Verification items for the finished model (mm, model axes). Round coordinates to 2 decimals unless told otherwise and drop trailing zeros. Loops run counter-clockwise (first coordinate to the right, second up) from the corner with the lowest first, then second, coordinate; pieces in that order, holes last. Notation, with made-up numbers: (-3, 4.25) -> (45, 4.25) arc R22 ccw to (45, 10.25) -> close; hole circle Ø9 at (-17.75, -30.75). An arc over 180 degrees is marked (long way). Use CSV: the item, a comma, the result in double quotes. Start each with the question number.
Autodesk Inventor part; units mm, degrees
ref_plane "YZ Plane" through (0, 0, 0) normal (1, 0, 0) x (0, 1, 0)
ref_plane "XZ Plane" through (0, 0, 0) normal (0, 1, 0) x (-1, 0, 0)
ref_plane "XY Plane" through (0, 0, 0) normal (0, 0, 1) x (1, 0, 0)
sketch "Sketch1" plane through (0, 0, 0) normal (0, 1, 0) x (-1, 0, 0)
  arc A0 (-2.75, 2.165064) -> (2.75, 2.165064) centre (0, 0) ccw
  line L0 (-1.9, 14.1) -> (-2.75, 2.165064)
  line L1 (1.898718, 14.098684) -> (2.75, 2.165064)
  arc A1 (1.898718, 14.098684) -> (-1.9, 14.1) centre (-0.000658, 14.05) ccw
  circle A2 centre (0, 0) radius 0.5
  line L2 (0, 0) -> (0, -10) construction
  line L3 (0, 30) -> (0, 0) construction
  arc A3 (-7.653502, 3.697825) -> (7.653343, 3.698154) centre (0, 0) ccw
  line L4 (7.653343, 3.698154) -> (6.891627, 14.376202)
  arc A4 (6.891627, 14.376202) -> (-6.892842, 14.378331) centre (-0.000658, 14.05) ccw
  line L5 (-6.892842, 14.378331) -> (-7.653502, 3.697825)
  line L6 (10, 0) -> (-10, 0)
  line L7 (-10, 0) -> (-10, 30)
  line L8 (-10, 30) -> (10, 30)
  line L9 (10, 30) -> (10, 0)
  point P0 (-8.5, 0)
  point P1 (8.5, 0)
  dimension "d0" = 1
  dimension "d9" = 1.9
  dimension "d11" = 3.5
  dimension "d34" = 10
  dimension "d42" = 5
  dimension "d43" = 20
  dimension "d44" = 30
sketch "Sketch1 outline for Extrusion6" plane through (0, 0, 0) normal (0, 1, 0) x (-1, 0, 0)
  arc A0 (-8.5, 0) -> (8.5, 0) centre (0, 0) ccw
  line L0 (-10, 0) -> (-8.5, 0)
  line L1 (8.5, 0) -> (10, 0)
  line L2 (-10, 30) -> (-10, 0)
  line L3 (10, 0) -> (10, 30)
  line L4 (10, 30) -> (-10, 30)
  arc A1 (2.75, 2.165064) -> (-2.75, 2.165064) centre (0, 0) cw
  line L5 (1.898718, 14.098684) -> (2.75, 2.165064)
  arc A2 (-1.9, 14.1) -> (1.898718, 14.098684) centre (-0.000658, 14.05) cw
  line L6 (-2.75, 2.165064) -> (-1.9, 14.1)
extrude "Extrusion6" add sketch "Sketch1 outline for Extrusion6" along normal blind 8
sketch "Sketch7" plane through (0, 0, 0) normal (0, -1, 0) x (1, 0, 0)
  arc A0 (-8.5, 0) -> (8.5, 0) centre (0, 0) ccw
  line L0 (10, 30) -> (10, 0)
  line L1 (-10, 0) -> (-10, 30)
  line L2 (-10, 0) -> (-10, 30)
  line L3 (-10, 0) -> (-7.225, -4.477653)
  line L4 (10, 0) -> (7.225, -4.477653)
  line L5 (8.5, 0) -> (10, 0)
  line L6 (-8.5, 0) -> (-10, 0)
  line L7 (-8.5, 0) -> (-10, 0)
sketch "Sketch7 outline for Extrusion7" plane through (0, 0, 0) normal (0, -1, 0) x (1, 0, 0)
  line L0 (-8.5, 0) -> (-10, 0)
  arc A0 (-7.225, -4.477653) -> (-8.5, 0) centre (0, 0) cw
  line L1 (-10, 0) -> (-7.225, -4.477653)
  line L2 (10, 0) -> (8.5, 0)
  line L3 (7.225, -4.477653) -> (10, 0)
  arc A1 (8.5, 0) -> (7.225, -4.477653) centre (0, 0) cw
extrude "Extrusion7" add sketch "Sketch7 outline for Extrusion7" against normal blind 8
sketch "Sketch8" plane through (0, 0, 0) normal (0, -1, 0) x (1, 0, 0)
  line L0 (-10, 0) -> (-7.225, -4.477653)
  arc A0 (-7.225, -4.477653) -> (7.225, -4.477653) centre (0, 0) ccw
  line L1 (7.225, -4.477653) -> (10, 0)
  line L2 (10, 30) -> (10, 0)
  line L3 (-10, 30) -> (10, 30)
  line L4 (-10, 0) -> (-10, 30)
  arc A1 (-2.75, 2.165064) -> (2.75, 2.165064) centre (0, 0) ccw
  line L5 (-1.898718, 14.098684) -> (-2.75, 2.165064)
  arc A2 (1.9, 14.1) -> (-1.898718, 14.098684) centre (0.000658, 14.05) ccw
  line L6 (2.75, 2.165064) -> (1.9, 14.1)
  circle A3 centre (0, 20) radius 10
  line L7 (10, 30) -> (10, 1.423737)
  line L8 (-10, 30) -> (10, 30)
  point P0 (-10, 20)
  point P1 (0, 30)
  point P2 (10, 20)
  point P3 (2.174951, 10.239386)
  point P4 (-2.174035, 10.239182)
  dimension "d50" = 20
sketch "Sketch8 outline for Extrusion8" plane through (0, 0, 0) normal (0, -1, 0) x (1, 0, 0)
  arc A0 (-10, 20) -> (0, 30) centre (0, 20) cw
  line L0 (-10, 30) -> (-10, 20)
  line L1 (0, 30) -> (-10, 30)
  arc A1 (0, 30) -> (10, 20) centre (0, 20) cw
  line L2 (10, 30) -> (0, 30)
  line L3 (10, 20) -> (10, 30)
extrude "Extrusion8" cut sketch "Sketch8 outline for Extrusion8" against normal through all
sketch "Sketch9" plane through (0, 8, 0) normal (0, 1, 0) x (1, 0, 0)
  arc A0 (-10, -20) -> (10, -20) centre (0, -20) ccw
  line L0 (-10, 0) -> (-10, -20)
  arc A1 (-9.25, 1.210176) -> (-10, -1.423737) centre (-5, -1.423737) ccw
  line L1 (-7.225, 4.477653) -> (-10, 0)
  arc A2 (7.225, 4.477653) -> (-7.225, 4.477653) centre (0, 0) ccw
  line L2 (10, 0) -> (7.225, 4.477653)
  arc A3 (10, -1.423737) -> (9.25, 1.210176) centre (5, -1.423737) ccw
  line L3 (10, -20) -> (10, 0)
sketch "Sketch9 outline for Extrusion9" plane through (0, 8, 0) normal (0, 1, 0) x (1, 0, 0)
  arc A0 (-10, -20) -> (10, -20) centre (0, -20) ccw
  line L0 (-10, -1.423737) -> (-10, -20)
  arc A1 (-9.25, 1.210176) -> (-10, -1.423737) centre (-5, -1.423737) ccw
  line L1 (-7.225, 4.477653) -> (-9.25, 1.210176)
  arc A2 (7.225, 4.477653) -> (-7.225, 4.477653) centre (0, 0) ccw
  line L2 (9.25, 1.210176) -> (7.225, 4.477653)
  arc A3 (10, -1.423737) -> (9.25, 1.210176) centre (5, -1.423737) ccw
  line L3 (10, -20) -> (10, -1.423737)
extrude "Extrusion9" add sketch "Sketch9 outline for Extrusion9" against normal blind 5
sketch "Sketch10" plane through (0, 0, 0) normal (0, -1, 0) x (1, 0, 0)
  line L0 (10, 20) -> (10, 0)
  line L1 (0, 0) -> (10, 0)
  line L2 (10, 0) -> (10, 65)
  line L3 (10, 65) -> (0, 65)
  line L4 (0, 65) -> (0, 0) construction
  line L5 (-10, 0) -> (-10, 20)
  line L6 (0, 0) -> (-10, 0)
  line L7 (-10, 0) -> (-10, 65)
  line L8 (-10, 65) -> (0, 65)
  dimension "d55" = 65
sketch "Sketch10 outline for Extrusion10" plane through (0, 0, 0) normal (0, -1, 0) x (1, 0, 0)
  line L0 (-10, 0) -> (0, 0)
  line L1 (-10, 20) -> (-10, 0)
  line L2 (-10, 65) -> (-10, 20)
  line L3 (0, 65) -> (-10, 65)
  line L4 (10, 65) -> (0, 65)
  line L5 (10, 20) -> (10, 65)
  line L6 (10, 0) -> (10, 20)
  line L7 (0, 0) -> (10, 0)
extrude "Extrusion10" add sketch "Sketch10 outline for Extrusion10" against normal blind 8
sketch "Sketch8 outline for Extrusion11" plane through (0, 0, 0) normal (0, -1, 0) x (1, 0, 0)
  arc A0 (-2.75, 2.165064) -> (2.75, 2.165064) centre (0, 0) ccw
  line L0 (-2.174035, 10.239182) -> (-2.75, 2.165064)
  arc A1 (2.174951, 10.239386) -> (-2.174035, 10.239182) centre (0, 20) cw
  line L1 (2.75, 2.165064) -> (2.174951, 10.239386)
extrude "Extrusion11" cut sketch "Sketch8 outline for Extrusion11" against normal blind 3
sketch "Sketch8 outline for Extrusion12" plane through (0, 0, 0) normal (0, -1, 0) x (1, 0, 0)
  arc A0 (1.9, 14.1) -> (-1.898718, 14.098684) centre (0.000658, 14.05) ccw
  line L0 (2.174951, 10.239386) -> (1.9, 14.1)
  arc A1 (-2.174035, 10.239182) -> (2.174951, 10.239386) centre (0, 20) ccw
  line L1 (-1.898718, 14.098684) -> (-2.174035, 10.239182)
extrude "Extrusion12" cut sketch "Sketch8 outline for Extrusion12" against normal blind 3
properties part number "Servo_Shaft_select_V2_3DPrint"
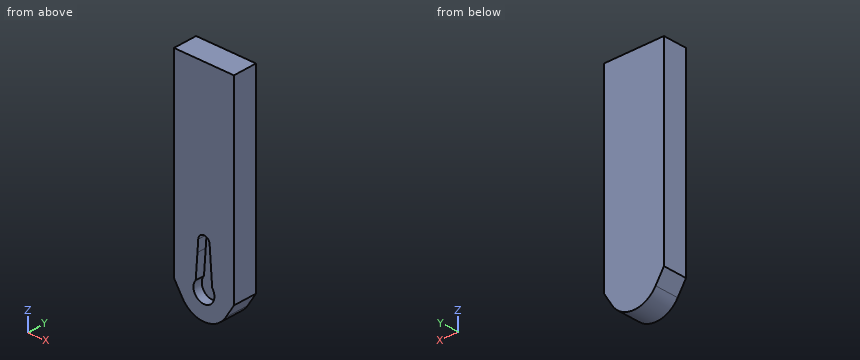
Q1. Depth check by flat-ended pin: pin 1 Ø2 at (x, z) = (1, 10.5) entering from -Y. Enter the tip coordinate at first touch or a pass-through.
Q2. Thickness scan on L1, parallel to X at y = 1.5, z = 0; L2, parallel to Y at x = -3, z = 0; L3, parallel to X at y = 2.75, z = 10. Record the ranges inside material, lowest first. Write a range as from..to.
Q3. Cross-section at C-C (y = 6.5). Record the boundary of the cut face in (x, z) (3 decimals), and give its area (3 significant figures).
Q4. Cross-section at A-A (y = 0.75). Record the boundary of the cut face in (x, z) (3 decimals).
Q5. Cross-section at B-B (x = 0). Record the boundary of the cut face in (y, z), and give its area (3 significant figures).
Answer list:
1,pin 1,"stops at y = 3"
2,L1,"x = -10..-3.5, 3.5..10"
2,L2,"y = 3..8"
2,L3,"x = -10..-2.19, 2.19..10"
3,outline,"(-10, 0) -> (-7.225, -4.478) arc R8.5 ccw to (7.225, -4.478) -> (10, 0) -> (10, 65) -> (-10, 65) -> close"
3,area,"1,420 mm2"
4,outline,"(-10, 0) -> (-7.225, -4.478) arc R8.5 ccw to (7.225, -4.478) -> (10, 0) -> (10, 65) -> (-10, 65) -> close; hole (-2.75, 2.165) arc R3.5 ccw (long way) to (2.75, 2.165) -> (1.9, 14.1) arc R1.9 ccw to (-1.899, 14.099) -> (-2.174, 10.239) -> close"
5,outline,"(0, -8.5) -> (8, -8.5) -> (8, 65) -> (0, 65) -> (0, 15.95) -> (3, 15.95) -> (3, -3.5) -> (0, -3.5) -> close"
5,area,"530 mm2"
